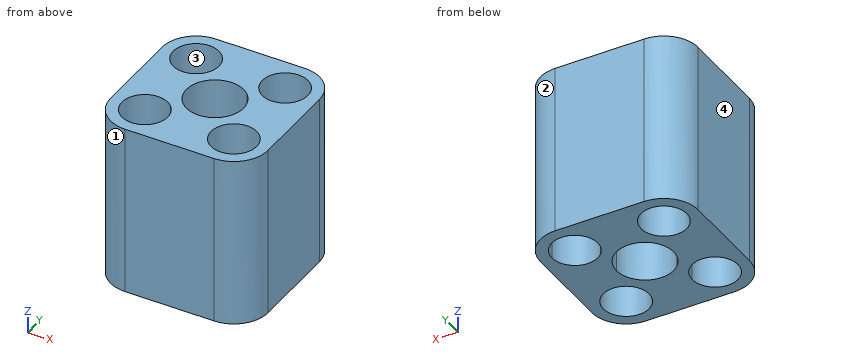
from build123d import *

# Parameters (mm, degrees)
F0_R     = 2
F1_DEPTH = 15


with BuildPart() as f1:
    # F0 (on Top) → F1 (new body)
    with BuildSketch(Plane.XY):
        with BuildLine():
            ThreePointArc((-2.474874, -2.474874), (-5.736846, -4.654454), (-1.889087, -3.889087))
            ThreePointArc((-1.889087, -3.889087), (-2.041328, -3.12372), (-2.474874, -2.474874))
        make_face()
        with BuildLine():
            ThreePointArc((5.889087, 3.889087), (3.12372, 5.736846), (2.474874, 2.474874))
            ThreePointArc((2.474874, 2.474874), (4.654454, 2.041328), (5.889087, 3.889087))
        make_face()
        with BuildLine():
            ThreePointArc((-6.889087, -3.889087), (-6.010408, -6.010408), (-3.889087, -6.889087))
            Line((-3.889087, -6.889087), (3.889087, -6.889087))
            ThreePointArc((3.889087, -6.889087), (6.010408, -6.010408), (6.889087, -3.889087))
            Line((6.889087, -3.889087), (6.889087, 3.889087))
            ThreePointArc((6.889087, 3.889087), (6.010408, 6.010408), (3.889087, 6.889087))
            Line((3.889087, 6.889087), (-3.889087, 6.889087))
            ThreePointArc((-3.889087, 6.889087), (-6.010408, 6.010408), (-6.889087, 3.889087))
            Line((-6.889087, 3.889087), (-6.889087, -3.889087))
        make_face()
        with BuildLine():
            ThreePointArc((-2.474874, -2.474874), (-2.041328, -3.12372), (-1.889087, -3.889087))
            ThreePointArc((-1.889087, -3.889087), (-5.736846, -4.654454), (-2.474874, -2.474874))
        make_face(mode=Mode.SUBTRACT)
        with Locations((3.889087, -3.889087)):
            Circle(F0_R, mode=Mode.SUBTRACT)
        with Locations((-3.889087, 3.889087)):
            Circle(F0_R, mode=Mode.SUBTRACT)
        with BuildLine():
            ThreePointArc((2.5, 0), (0.956709, -2.309699), (-1.767767, -1.767767))
            ThreePointArc((-1.767767, -1.767767), (-1.767767, 1.767767), (1.767767, 1.767767))
            ThreePointArc((1.767767, 1.767767), (2.309699, 0.956709), (2.5, 0))
        make_face(mode=Mode.SUBTRACT)
        with BuildLine():
            ThreePointArc((5.889087, 3.889087), (4.654454, 2.041328), (2.474874, 2.474874))
            ThreePointArc((2.474874, 2.474874), (3.12372, 5.736846), (5.889087, 3.889087))
        make_face(mode=Mode.SUBTRACT)
    extrude(amount=F1_DEPTH)


solid = f1.part
The listing builds one solid part. Answer for the finished solid, in the listing's coordinates (mm). Face numbers are marked on the shaded views. Give positions to 0.01 mm unless a question says otherwise; leave off trailing zeros. Loops run counter-clockwise (first coordinate to the right, second up) from the corner with the lowest first, then second, coordinate; pieces in that order, holes last.
Item 1: Each of these flat-tipped pins is pushed along its axis until it touches: pin 1 Ø2 at (y, z) = (-5, 13) entering from -X; pin 2 Ø3.5 at (x, y) = (-3.89, 3.89) entering from -Z. Where does it stop, or does it pass through?
Derived:
pin 1: stops at x = -6.89
pin 2: passes through
Item 2: Determine the mould class of the marked faces 1, 2, 3 and 4 for opening direction Y: +Y half, -Y half, draft (parallel to the pull), parting line (faces both ways), or undercut.
Derived:
face 1: -Y half
face 2: +Y half
face 3: undercut
face 4: draft
Item 3: A cutting plane is placed at B-B (y = 4.5). Give the vertices of the cut face in (x, z), then the cut area to 3 significant figures.
Derived:
outline: (-6.83, 0) - (-5.79, 0) - (-5.79, 15) - (-6.83, 15) - close; (-1.98, 0) - (1.98, 0) - (1.98, 15) - (-1.98, 15) - close; (5.79, 0) - (6.83, 0) - (6.83, 15) - (5.79, 15) - close
area: 90.5 mm2
Item 4: A cutting plane is placed at C-C (z = 10). Give the vertices of the cut face in (x, y), then the cut area to 3 significant figures.
Derived:
outline: (-6.89, -3.89) arc R3 ccw to (-3.89, -6.89) - (3.89, -6.89) arc R3 ccw to (6.89, -3.89) - (6.89, 3.89) arc R3 ccw to (3.89, 6.89) - (-3.89, 6.89) arc R3 ccw to (-6.89, 3.89) - close; hole circle Ø4 at (-3.89, 3.89); hole (-2.47, -2.47) arc R2 ccw (long way) to (-1.89, -3.89) arc R2 ccw to start; hole (1.77, 1.77) arc R2.5 ccw (long way) to (2.5, 0) arc R2.5 ccw to start; hole circle Ø4 at (3.89, -3.89); hole circle Ø4 at (3.89, 3.89)
area: 112 mm2
Item 5: Find the intervals of material crossed by line 1 along Y through (x, z) = (4, 13.75); line 2 along X through (y, z) = (-3.75, 2.25); line 3 along X through (y, z) = (-3.25, 3), in increasing order.
Derived:
line 1: y = -6.89 to -5.89, -1.89 to 1.89, 5.89 to 6.89
line 2: x = -6.89 to -5.88, -1.89 to 1.89, 5.88 to 6.89
line 3: x = -6.89 to -5.78, -1.99 to 1.99, 5.78 to 6.89
Item 6: A cutting plane is placed at A-A (x = 0). Give the vertices of the cut face in (y, z), then the cut area to 3 significant figures.
Derived:
outline: (-6.89, 0) - (-2.5, 0) - (-2.5, 15) - (-6.89, 15) - close; (2.5, 0) - (6.89, 0) - (6.89, 15) - (2.5, 15) - close
area: 132 mm2
